```python
from build123d import *

# Parameters (mm, degrees)
F1_DEPTH = 48
F2_W     = 16
F2_H     = 6.5
F3_DEPTH = 11
F4_R     = 11
F5_DEPTH = 2
F6_R     = 2.25
F7_DEPTH = 25


with BuildPart() as f1:
    # F0 (on Top) → F1 (new body)
    with BuildSketch(Plane.XY):
        Polygon((16.15, 21.15), (-16.15, 21.15), (-21.15, 16.15), (-21.15, -16.15), (-16.15, -21.15), (16.15, -21.15), (21.15, -16.15), (21.15, 16.15), align=None)
    extrude(amount=F1_DEPTH)

    # F2 (on Top) → F3 (join)
    with BuildSketch(Plane.XY):
        with Locations((0, 24.4)):
            Rectangle(F2_W, F2_H)
    extrude(amount=F3_DEPTH)

    # F4 (on face) → F5 (join)
    with BuildSketch(Plane.XY.offset(48)):
        Circle(F4_R)
    extrude(amount=F5_DEPTH)

    # F6 (on face) → F7 (join)
    with BuildSketch(Plane.XY.offset(50)):
        Circle(F6_R)
    extrude(amount=F7_DEPTH)


solid = f1.part
```
Geometry: final body of the model. Coordinates: model frame, mm. A direction names the side the tool comes from. Coordinates: 2 decimals unless noted, no trailing zeros. Order: outer loops, then holes, each group sorted by start corner. A loop starts at its lowest first (then second) coordinate and runs counter-clockwise, first axis right, second up. Notation, with made-up numbers: M 55.25,27.25 L 61.25,27.25 A19 ccw 61.25,46.25 Z; hole C 89.25,67.25 d5. An arc over 180 degrees is marked long. Answer in a Markdown table with one row per item. Add a question column.
Q1. Section query D-D on y = 15. Return the cut outline in (x, z).
Q2. Section query B-B on x = 0. Return the cut outline in (y, z), and give its area (3 significant figures).
Q3. Section query A-A on y = 0. Return the cut outline in (x, z), and give its area (3 significant figures).
Q4. Line query: L1, parallel to Z at x = -3, y = -14.5; L2, parallel to Y at x = -5.5, z = 13; L3, parallel to Z at x = -6, y = 1.5. Output: solid intervals per line, ascending.
Q5. Contact query for flat-ended pins moving along their axis: P1, Ø5, axis at x = 2, y = 25.5, coming from the +Z side; P2, Ø12, axis at x = -17, z = 38.5, coming from the +Y side; P3, Ø7, axis at y = 24, z = 4, coming from the -X side. Output: stop coordinate, or through.
Q6. Section query C-C on z = 5. Return the cut outline in (x, y).
Q7. Reachability of faces 1 (the flat face through (0, 24, 11)), 2 (the flat face through (-8, 24, 5)), 3 (the flat face through (9, -9, 48)) from +Z, -Z, +X, -X, +Y, -Y: full face, straight path, thin tool, end or side. Return the list, or none.
Completed:
| question | item | result |
|---|---|---|
| 1 | outline | M -21.15,0 L 21.15,0 L 21.15,48 L -21.15,48 Z |
| 2 | outline | M -21.15,0 L 27.65,0 L 27.65,11 L 21.15,11 L 21.15,48 L 11,48 L 11,50 L 2.25,50 L 2.25,75 L -2.25,75 L -2.25,50 L -11,50 L -11,48 L -21.15,48 Z |
| 2 | area | 2,260 mm2 |
| 3 | outline | M -21.15,0 L 21.15,0 L 21.15,48 L 11,48 L 11,50 L 2.25,50 L 2.25,75 L -2.25,75 L -2.25,50 L -11,50 L -11,48 L -21.15,48 Z |
| 3 | area | 2,190 mm2 |
| 4 | L1 | z = 0 to 48 |
| 4 | L2 | y = -21.15 to 21.15 |
| 4 | L3 | z = 0 to 50 |
| 5 | P1 | stops at z = 11 |
| 5 | P2 | stops at y = 21.15 |
| 5 | P3 | stops at x = -16.8 |
| 6 | outline | M -21.15,-16.15 L -16.15,-21.15 L 16.15,-21.15 L 21.15,-16.15 L 21.15,16.15 L 16.15,21.15 L 8,21.15 L 8,27.65 L -8,27.65 L -8,21.15 L -16.15,21.15 L -21.15,16.15 Z |
| 7 | face 1 | +Z, +X, -X, +Y |
| 7 | face 2 | +Z, -Z, -X, +Y |
| 7 | face 3 | +Z |
